Source: CAD feature listing. Evaluate the final solid. Frame: model axes, mm. Give positions to 0.01 mm unless a question says otherwise; leave off trailing zeros. Order: outer loops, then holes, each group sorted by start corner. A loop starts at its lowest first (then second) coordinate and runs counter-clockwise, first axis right, second up. Notation, with made-up numbers: M 47,37.5 L 63,37.5 A8 ccw 63,46.5 Z; hole C 62,60.5 d7. An arc over 180 degrees is marked long. Answer as a JSON object with one key per item and string values. Group by question number.
1. Material intervals for L1, parallel to Z at x = 29, y = 2.5; L2, parallel to Z at x = -7, y = 3; L3, parallel to X at y = 2.8, z = 44.5, sorted ascending. Write a range as [from, to].
2. Section query C-C (y = 2.6). Count the separate pieces of the cut face and the enclosed holes in it, plus the area to 3 significant figures.
3. Section query B-B (z = -62). Output: boundary loops of the cut face in (x, y).
4. Section query A-A (x = 5.5). Output: boundary loops of the cut face in (y, z).
5. Pin query (flat end, axial travel): P1, Ø1.5, axis at y = 1.5, z = -73.5, coming from the +X side; P2, Ø11.5, axis at x = -88.39, z = 88.39, coming from the +Y side; P3, Ø1.7, axis at x = -89, z = -106, coming from the +Y side; P4, Ø1.5, axis at x = 92.5, y = 3, coming from the +Z side. Return the tip coordinate at first contact, or that it passes through.
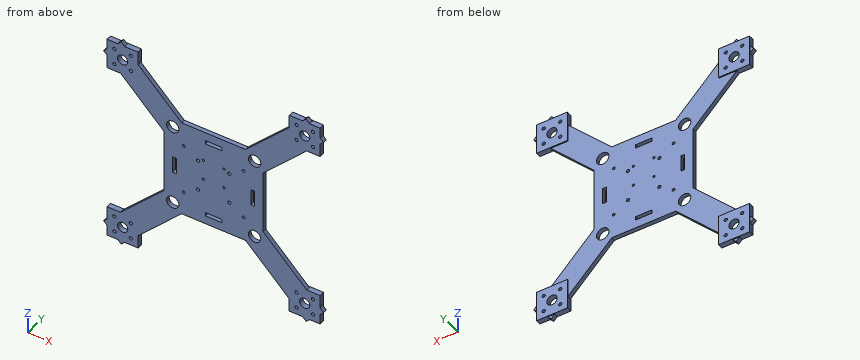
from build123d import *

# Parameters (mm, degrees)
SKETCH1_W            = 96
SKETCH1_H            = 96
CENTERDECK_DEPTH     = 4
ARM1_DEPTH           = 4
ARM2_DEPTH           = 4
ARM3_DEPTH           = 4
ARM4_DEPTH           = 4
SKETCH6_W            = 30
SKETCH6_H            = 30
MOTORPAD1_DEPTH      = 5
SKETCH7_W            = 30
SKETCH7_H            = 30
MOTORPAD2_DEPTH      = 5
SKETCH8_W            = 30
SKETCH8_H            = 30
MOTORPAD3_DEPTH      = 5
SKETCH9_W            = 30
SKETCH9_H            = 30
MOTORPAD4_DEPTH      = 5
SKETCH10_R           = 1.6
SKETCH10_R_2         = 5
MOTORHOLES1_DEPTH    = 152.082758778
SKETCH11_R           = 1.6
SKETCH11_R_2         = 5
MOTORHOLES2_DEPTH    = 152.082758778
SKETCH12_R           = 1.6
SKETCH12_R_2         = 5
MOTORHOLES3_DEPTH    = 152.082758778
SKETCH13_R           = 1.6
SKETCH13_R_2         = 5
MOTORHOLES4_DEPTH    = 152.082758778
SKETCH14_R           = 1.6
STACKHOLES_DEPTH     = 152.082758778
SKETCH15_R           = 1.35
PIHOLES_DEPTH        = 152.082758778
SKETCH16_W           = 3.5
SKETCH16_H           = 16
SKETCH16_W_2         = 16
SKETCH16_H_2         = 3.5
BATTSTRAPSLOTS_DEPTH = 152.082758778
SKETCH17_R           = 1.1
CAMERAHOLES_DEPTH    = 152.082758778
SKETCH18_R           = 6
ARMLIGHTENING_DEPTH  = 152.082758778


with BuildPart() as part:
    # Sketch1 → CenterDeck (new body)
    with BuildSketch(Plane(origin=(0, 0, 0), x_dir=(1, 0, 0), z_dir=(0, 1, 0))):
        Rectangle(SKETCH1_W, SKETCH1_H)
    extrude(amount=CENTERDECK_DEPTH)

    # Sketch2 → Arm1 (add)
    with BuildSketch(Plane(origin=(0, 0, 0), x_dir=(1, 0, 0), z_dir=(0, 1, 0))):
        Polygon((22.627416998, 39.597979746), (39.597979746, 22.627416998), (106.773123959, 89.802561211), (89.802561211, 106.773123959), align=None)
    extrude(amount=ARM1_DEPTH)

    # Sketch3 → Arm2 (add)
    with BuildSketch(Plane(origin=(0, 0, 0), x_dir=(1, 0, 0), z_dir=(0, 1, 0))):
        Polygon((39.597979746, -22.627416998), (22.627416998, -39.597979746), (89.802561211, -106.773123959), (106.773123959, -89.802561211), align=None)
    extrude(amount=ARM2_DEPTH)

    # Sketch4 → Arm3 (add)
    with BuildSketch(Plane(origin=(0, 0, 0), x_dir=(1, 0, 0), z_dir=(0, 1, 0))):
        Polygon((-39.597979746, 22.627416998), (-22.627416998, 39.597979746), (-89.802561211, 106.773123959), (-106.773123959, 89.802561211), align=None)
    extrude(amount=ARM3_DEPTH)

    # Sketch5 → Arm4 (add)
    with BuildSketch(Plane(origin=(0, 0, 0), x_dir=(1, 0, 0), z_dir=(0, 1, 0))):
        Polygon((-22.627416998, -39.597979746), (-39.597979746, -22.627416998), (-106.773123959, -89.802561211), (-89.802561211, -106.773123959), align=None)
    extrude(amount=ARM4_DEPTH)

    # Sketch6 → MotorPad1 (add)
    with BuildSketch(Plane(origin=(0, 0, 0), x_dir=(1, 0, 0), z_dir=(0, 1, 0))):
        with Locations((88.388347648, 88.388347648)):
            Rectangle(SKETCH6_W, SKETCH6_H)
    extrude(amount=MOTORPAD1_DEPTH)

    # Sketch7 → MotorPad2 (add)
    with BuildSketch(Plane(origin=(0, 0, 0), x_dir=(1, 0, 0), z_dir=(0, 1, 0))):
        with Locations((88.388347648, -88.388347648)):
            Rectangle(SKETCH7_W, SKETCH7_H)
    extrude(amount=MOTORPAD2_DEPTH)

    # Sketch8 → MotorPad3 (add)
    with BuildSketch(Plane(origin=(0, 0, 0), x_dir=(1, 0, 0), z_dir=(0, 1, 0))):
        with Locations((-88.388347648, 88.388347648)):
            Rectangle(SKETCH8_W, SKETCH8_H)
    extrude(amount=MOTORPAD3_DEPTH)

    # Sketch9 → MotorPad4 (add)
    with BuildSketch(Plane(origin=(0, 0, 0), x_dir=(1, 0, 0), z_dir=(0, 1, 0))):
        with Locations((-88.388347648, -88.388347648)):
            Rectangle(SKETCH9_W, SKETCH9_H)
    extrude(amount=MOTORPAD4_DEPTH)

    # Sketch10 → MotorHoles1 (cut, through all)
    with BuildSketch(Plane(origin=(0, 0, 0), x_dir=(1, 0, 0), z_dir=(0, 1, 0))):
        with Locations(Location((96.388347648, 96.388347648, 0), (0, 0, 270))):
            Circle(SKETCH10_R)
        with Locations(Location((96.388347648, 80.388347648, 0), (0, 0, 270))):
            Circle(SKETCH10_R)
        with Locations(Location((80.388347648, 96.388347648, 0), (0, 0, 270))):
            Circle(SKETCH10_R)
        with Locations(Location((80.388347648, 80.388347648, 0), (0, 0, 270))):
            Circle(SKETCH10_R)
        with Locations(Location((88.388347648, 88.388347648, 0), (0, 0, 270))):
            Circle(SKETCH10_R_2)
    extrude(amount=MOTORHOLES1_DEPTH, mode=Mode.SUBTRACT)

    # Sketch11 → MotorHoles2 (cut, through all)
    with BuildSketch(Plane(origin=(0, 0, 0), x_dir=(1, 0, 0), z_dir=(0, 1, 0))):
        with Locations(Location((96.388347648, -80.388347648, 0), (0, 0, 270))):
            Circle(SKETCH11_R)
        with Locations(Location((96.388347648, -96.388347648, 0), (0, 0, 270))):
            Circle(SKETCH11_R)
        with Locations(Location((80.388347648, -80.388347648, 0), (0, 0, 270))):
            Circle(SKETCH11_R)
        with Locations(Location((80.388347648, -96.388347648, 0), (0, 0, 270))):
            Circle(SKETCH11_R)
        with Locations(Location((88.388347648, -88.388347648, 0), (0, 0, 270))):
            Circle(SKETCH11_R_2)
    extrude(amount=MOTORHOLES2_DEPTH, mode=Mode.SUBTRACT)

    # Sketch12 → MotorHoles3 (cut, through all)
    with BuildSketch(Plane(origin=(0, 0, 0), x_dir=(1, 0, 0), z_dir=(0, 1, 0))):
        with Locations(Location((-80.388347648, 96.388347648, 0), (0, 0, 270))):
            Circle(SKETCH12_R)
        with Locations(Location((-80.388347648, 80.388347648, 0), (0, 0, 270))):
            Circle(SKETCH12_R)
        with Locations(Location((-96.388347648, 96.388347648, 0), (0, 0, 270))):
            Circle(SKETCH12_R)
        with Locations(Location((-96.388347648, 80.388347648, 0), (0, 0, 270))):
            Circle(SKETCH12_R)
        with Locations(Location((-88.388347648, 88.388347648, 0), (0, 0, 270))):
            Circle(SKETCH12_R_2)
    extrude(amount=MOTORHOLES3_DEPTH, mode=Mode.SUBTRACT)

    # Sketch13 → MotorHoles4 (cut, through all)
    with BuildSketch(Plane(origin=(0, 0, 0), x_dir=(1, 0, 0), z_dir=(0, 1, 0))):
        with Locations(Location((-80.388347648, -80.388347648, 0), (0, 0, 270))):
            Circle(SKETCH13_R)
        with Locations(Location((-80.388347648, -96.388347648, 0), (0, 0, 270))):
            Circle(SKETCH13_R)
        with Locations(Location((-96.388347648, -80.388347648, 0), (0, 0, 270))):
            Circle(SKETCH13_R)
        with Locations(Location((-96.388347648, -96.388347648, 0), (0, 0, 270))):
            Circle(SKETCH13_R)
        with Locations(Location((-88.388347648, -88.388347648, 0), (0, 0, 270))):
            Circle(SKETCH13_R_2)
    extrude(amount=MOTORHOLES4_DEPTH, mode=Mode.SUBTRACT)

    # Sketch14 → StackHoles (cut, through all)
    with BuildSketch(Plane(origin=(0, 0, 0), x_dir=(1, 0, 0), z_dir=(0, 1, 0))):
        with Locations(Location((15.25, 15.25, 0), (0, 0, 270))):
            Circle(SKETCH14_R)
        with Locations(Location((15.25, -15.25, 0), (0, 0, 270))):
            Circle(SKETCH14_R)
        with Locations(Location((-15.25, 15.25, 0), (0, 0, 270))):
            Circle(SKETCH14_R)
        with Locations(Location((-15.25, -15.25, 0), (0, 0, 270))):
            Circle(SKETCH14_R)
    extrude(amount=STACKHOLES_DEPTH, mode=Mode.SUBTRACT)

    # Sketch15 → PiHoles (cut, through all)
    with BuildSketch(Plane(origin=(0, 0, 0), x_dir=(1, 0, 0), z_dir=(0, 1, 0))):
        with Locations(Location((29, 24.5, 0), (0, 0, 270))):
            Circle(SKETCH15_R)
        with Locations(Location((29, -24.5, 0), (0, 0, 270))):
            Circle(SKETCH15_R)
        with Locations(Location((-29, 24.5, 0), (0, 0, 270))):
            Circle(SKETCH15_R)
        with Locations(Location((-29, -24.5, 0), (0, 0, 270))):
            Circle(SKETCH15_R)
    extrude(amount=PIHOLES_DEPTH, mode=Mode.SUBTRACT)

    # Sketch16 → BattStrapSlots (cut, through all)
    with BuildSketch(Plane(origin=(0, 0, 0), x_dir=(1, 0, 0), z_dir=(0, 1, 0))):
        with Locations((-38, 0)):
            Rectangle(SKETCH16_W, SKETCH16_H)
        with Locations((38, 0)):
            Rectangle(SKETCH16_W, SKETCH16_H)
        with Locations((0, 38)):
            Rectangle(SKETCH16_W_2, SKETCH16_H_2)
        with Locations((0, -38)):
            Rectangle(SKETCH16_W_2, SKETCH16_H_2)
    extrude(amount=BATTSTRAPSLOTS_DEPTH, mode=Mode.SUBTRACT)

    # Sketch17 → CameraHoles (cut, through all)
    with BuildSketch(Plane(origin=(0, 0, 0), x_dir=(1, 0, 0), z_dir=(0, 1, 0))):
        with Locations(Location((10, 2, 0), (0, 0, 270))):
            Circle(SKETCH17_R)
        with Locations(Location((10, -18, 0), (0, 0, 270))):
            Circle(SKETCH17_R)
        with Locations(Location((-10, 2, 0), (0, 0, 270))):
            Circle(SKETCH17_R)
        with Locations(Location((-10, -18, 0), (0, 0, 270))):
            Circle(SKETCH17_R)
    extrude(amount=CAMERAHOLES_DEPTH, mode=Mode.SUBTRACT)

    # Sketch18 → ArmLightening (cut, through all)
    with BuildSketch(Plane(origin=(0, 0, 0), x_dir=(1, 0, 0), z_dir=(0, 1, 0))):
        with Locations(Location((39.774756442, 39.774756442, 0), (0, 0, 270))):
            Circle(SKETCH18_R)
        with Locations(Location((39.774756442, -39.774756442, 0), (0, 0, 270))):
            Circle(SKETCH18_R)
        with Locations(Location((-39.774756442, 39.774756442, 0), (0, 0, 270))):
            Circle(SKETCH18_R)
        with Locations(Location((-39.774756442, -39.774756442, 0), (0, 0, 270))):
            Circle(SKETCH18_R)
    extrude(amount=ARMLIGHTENING_DEPTH, mode=Mode.SUBTRACT)


solid = part.part
Answer sheet:
{
 "1": {"L1": "[-48, -25.85], [-23.15, 23.15], [25.85, 48]", "L2": "[-48, -39.75], [-36.25, 36.25], [39.75, 48]", "L3": "[-61.47, -43.47], [-36.08, 36.08], [43.47, 61.47]"},
 "2": {"separate pieces": "1", "enclosed holes": "40", "area": "16,300 mm^2"},
 "3": {"outline": "M -78.97,0 L -45.03,0 L -45.03,4 L -78.97,4 Z; M 45.03,0 L 78.97,0 L 78.97,4 L 45.03,4 Z"},
 "4": {"outline": "M 0,-48 L 4,-48 L 4,-39.75 L 0,-39.75 Z; M 0,-36.25 L 4,-36.25 L 4,36.25 L 0,36.25 Z; M 0,39.75 L 4,39.75 L 4,48 L 0,48 Z"},
 "5": {"P1": "x = 103.39", "P2": "y = 5", "P3": "y = 4", "P4": "z = 104.83"}
}
